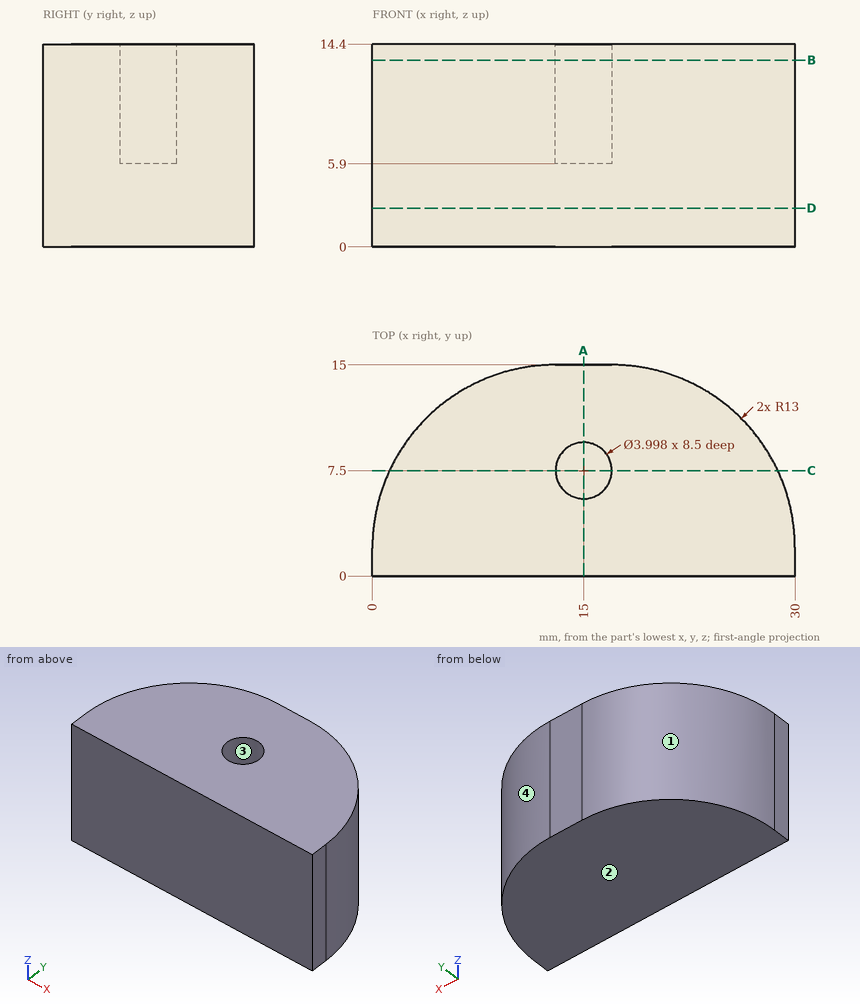
Verification items for this drawing (mm, ordinates from the low corner). Round coordinates to 2 decimals unless told otherwise and drop trailing zeros. Write each loop counter-clockwise with the first axis right and the second up, starting at its lowest first coordinate (ties: lowest second). Pieces come first, ordered by that corner, then holes. Notation, with made-up numbers: (46, -7) - (64, -7) arc R33 ccw to (64, 30) - close; hole circle Ø6 at (-6.75, -30). An arc over 180 degrees is marked (long way). One line per item, written item: value.
1. Scan lines: L1, parallel to Y at x = 15, z = 12.75; L2, parallel to X at y = 7.25, z = 8.75 (1 decimal); L3, parallel to Z at x = 14, y = 6. Record each from-to range of solid material in increasing order.
The answers:
L1: y = 0 to 5.5, 9.5 to 15
L2: x = 1.1 to 13, 17 to 28.9
L3: z = 0 to 5.9
2. Cross-section at A-A on x = 15. Record the boundary of the cut face in (y, z).
The answers:
outline: (0, 0) - (15, 0) - (15, 14.4) - (9.5, 14.4) - (9.5, 5.9) - (5.5, 5.9) - (5.5, 14.4) - (0, 14.4) - close
3. Cross-section at B-B on z = 13.25. Record the boundary of the cut face in (x, y), and give its area (3 significant figures).
The answers:
outline: (0, 0) - (30, 0) - (30, 2) arc R13 ccw to (17, 15) - (13, 15) arc R13 ccw to (0, 2) - close; hole circle Ø4 at (15, 7.5)
area: 365 mm^2
4. Cross-section at D-D on z = 2.75. Record the boundary of the cut face in (x, y).
The answers:
outline: (0, 0) - (30, 0) - (30, 2) arc R13 ccw to (17, 15) - (13, 15) arc R13 ccw to (0, 2) - close
5. Cross-section at C-C on y = 7.5. Record the boundary of the cut face in (x, z).
The answers:
outline: (1.22, 0) - (28.78, 0) - (28.78, 14.4) - (17, 14.4) - (17, 5.9) - (13, 5.9) - (13, 14.4) - (1.22, 14.4) - close
6. Mould release check, pull along X, two halves, no side actions. Record for the marked faces 1, 2, 3 and 4: released by +X, released by -X, zero draft, split by the parting line, or undercut.
The answers:
face 1: released by -X
face 2: zero draft
face 3: undercut
face 4: released by +X
7. Depth check by flat-ended pin: pin 1 Ø5 at (y, z) = (6, 4.5) entering from -X; pin 2 Ø1.5 at (y, z) = (8, 5.5) entering from +X; pin 3 Ø2 at (y, z) = (10, 10) entering from +X (1 decimal). Enter the tip coordinate at first touch or a pass-through.
The answers:
pin 1: stops at x = 0.09
pin 2: stops at x = 28.89
pin 3: stops at x = 28
